Could you check a few things on this drawing? It's one solid part, dimensions in mm from its lowest x, y, z. Coordinates: 2 decimals unless noted, no trailing zeros. Loops run counter-clockwise (first coordinate to the right, second up) from the corner with the lowest first, then second, coordinate; pieces in that order, holes last. Notation, with made-up numbers: (-36, 20.25) -> (2, 20.25) arc R8 cw to (2, 32.25) -> close; hole circle Ø10 at (68, 10.25). An arc over 180 degrees is marked (long way). One line per question, with ' | ' between items.
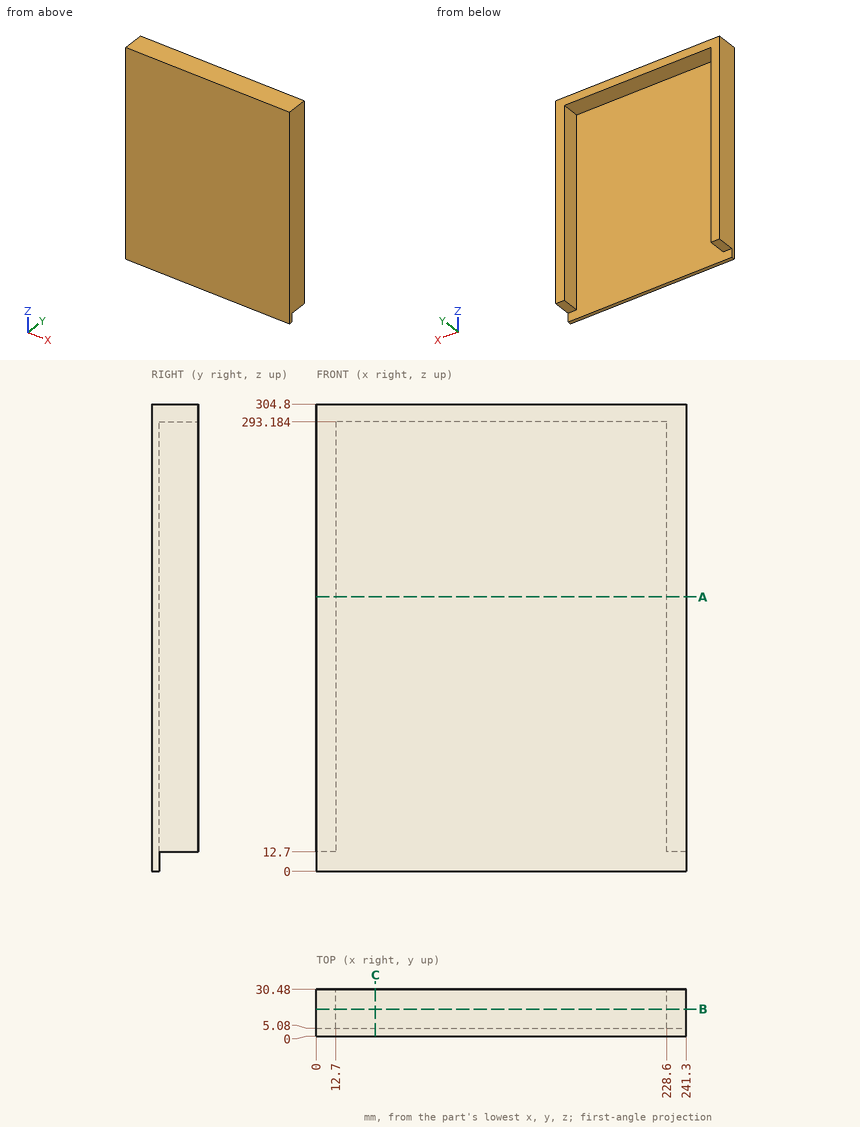
1) I need wall thicknesses on line 1 along X through (y, z) = (27, 87.5); line 2 along Y through (x, z) = (223, 125); line 3 along Z through (x, y) = (78, 6). Which ranges of each line are inside material? Lowest first, please. Write a range as from..to.
Data:
line 1: 0..12.7, 228.6..241.3 | line 2: 0..5.08 | line 3: 293.18..304.8
2) I'm going to push flat-ended pins straight in: pin 1 Ø4 at (x, z) = (169.5, 95.5) entering from +Y; pin 2 Ø12 at (x, y) = (200.5, 18.5) entering from -Z; pin 3 Ø12 at (y, z) = (9, 104.5) entering from -X; pin 4 Ø4 at (x, y) = (6.5, 24) entering from -Z. Where does each tip first touch, or does it pass through?
Data:
pin 1: y = 5.08 | pin 2: z = 293.18 | pin 3: x = 0 | pin 4: z = 12.7
3) If we section it at B-B on y = 17.5: Please give me the cut outline in (x, z), and give its area (3 significant figures).
Data:
outline: (0, 12.7) -> (12.7, 12.7) -> (12.7, 293.18) -> (228.6, 293.18) -> (228.6, 12.7) -> (241.3, 12.7) -> (241.3, 304.8) -> (0, 304.8) -> close | area: 9,930 mm²
4) If we section it at A-A on z = 179: Please give me the cut outline in (x, y), and give its area (3 significant figures).
Data:
outline: (0, 0) -> (241.3, 0) -> (241.3, 30.48) -> (228.6, 30.48) -> (228.6, 5.08) -> (12.7, 5.08) -> (12.7, 30.48) -> (0, 30.48) -> close | area: 1,870 mm²
5) If we section it at C-C on x = 38.5: Please give me the cut outline in (y, z).
Data:
outline: (0, 0) -> (5.08, 0) -> (5.08, 293.18) -> (30.48, 293.18) -> (30.48, 304.8) -> (0, 304.8) -> close
